The model under review builds one solid part; all positions refer to its coordinate system, in mm. A direction names the side the tool comes from. Coordinates: 2 decimals unless noted, no trailing zeros. Order: outer loops, then holes, each group sorted by start corner. A loop starts at its lowest first (then second) coordinate and runs counter-clockwise, first axis right, second up. Notation, with made-up numbers: (18, 26.25) -> (47, 26.25) arc R11 ccw to (47, 40.25) -> close; hole circle Ø11 at (69.5, 68). An arc over 180 degrees is marked (long way). Put each result on its own line as item: value.
from build123d import *

# Parameters (mm, degrees)
F0_R      = 22.5780805595
F5_DEPTH  = 25.4
F6_W      = 9.525
F6_H      = 38.1
F7_DEPTH  = 19.05
F8_R      = 5.08
F9_W      = 9.525
F9_H      = 38.1
F10_DEPTH = 19.05
F11_W     = 38.1
F11_H     = 9.525
F12_DEPTH = 19.05
F14_R     = 5.08
F13_W     = 8.255
F13_H     = 19.05
F15_DEPTH = 19.05
F16_R     = 8.25499
F17_SIZE  = 1.5875


# Not quite as in the source:
# - a fillet or chamfer is up to 0.001 mm smaller than in the source, because OpenCascade refuses the exact size


with BuildPart() as f2:
    # F2: sweep along a path in F1
    with BuildLine(Plane.XZ) as f2_path:
        Line((0, 0), (57.7025674284, 65.8432990313))
    # F0 (on Top) → F2 (sweep)
    with BuildSketch(Plane.XY):
        with Locations((-2.6368375402, 0)):
            Circle(F0_R)
    sweep(path=f2_path.line)


with BuildPart() as f5:
    # F4 (on Top) → F5 (new body)
    with BuildSketch(Plane.XY):
        with BuildLine():
            Line((-31.75, -19.05), (31.75, -19.05))
            Line((31.75, -19.05), (31.75, 19.05))
            Line((31.75, 19.05), (12.7, 19.05))
            ThreePointArc((12.7, 19.05), (0, 6.35), (-12.7, 19.05))
            Line((-12.7, 19.05), (-31.75, 19.05))
            Line((-31.75, 19.05), (-31.75, -19.05))
        make_face()
    extrude(amount=F5_DEPTH)

    # F6 (on face) → F7 (cut)
    with BuildSketch(Plane.XY.offset(25.4)):
        with Locations((26.9875, 0)):
            Rectangle(F6_W, F6_H)
    extrude(amount=-F7_DEPTH, mode=Mode.SUBTRACT)

    # F8
    f8_edges = [f5.edges().sort_by_distance(p)[0] for p in [
        (31.75, 19.05, 3.175),
    ]]
    fillet(f8_edges, radius=F8_R)

    # F9 (on face) → F10 (cut)
    with BuildSketch(Plane.XY.offset(25.4)):
        with Locations((-26.9875, 0)):
            Rectangle(F9_W, F9_H)
    extrude(amount=-F10_DEPTH, mode=Mode.SUBTRACT)

    # F11 (on face) → F12 (cut)
    with BuildSketch(Plane.XY.offset(25.4)):
        with Locations((0, -14.2875)):
            Rectangle(F11_W, F11_H)
    extrude(amount=-F12_DEPTH, mode=Mode.SUBTRACT)

    # F14
    f14_edges = [f5.edges().sort_by_distance(p)[0] for p in [
        (-31.75, 19.05, 3.175),
    ]]
    fillet(f14_edges, radius=F14_R)

    # F13 (on face) → F15 (cut)
    with BuildSketch(Plane.XY.offset(25.4)):
        with Locations((-18.0975, 9.525)):
            Rectangle(F13_W, F13_H)
        with Locations((18.0975, 9.525)):
            Rectangle(F13_W, F13_H)
    extrude(amount=-F15_DEPTH, mode=Mode.SUBTRACT)

    # F16 (radius 8.255 in the source; OpenCascade refuses exactly that, so slightly less here)
    f16_edges = [f5.edges().sort_by_distance(p)[0] for p in [
        (-13.97, 0, 15.875),
        (13.97, 0, 15.875),
    ]]
    fillet(f16_edges, radius=F16_R)

    # F17
    f17_edges = [f5.edges().sort_by_distance(p)[0] for p in [
        (0, 6.35, 25.4),
        (0, -9.525, 25.4),
        (-19.05, -14.2875, 25.4),
        (19.05, -14.2875, 25.4),
    ]]
    chamfer(f17_edges, length=F17_SIZE)


solid = f5.part
Item 1: For pin 1 Ø8.5 at (x, z) = (-4.5, 15) entering from -Y (3 decimals); pin 2 Ø7.5 at (y, z) = (-13, 13) entering from +X (3 decimals); pin 3 Ø2 at (x, z) = (-3, 19) entering from +Y, all flat-tipped, find the tip position at first contact; note any pin that passes through.
Answers below:
pin 1: y = -9.525
pin 2: x = 22.225
pin 3: y = 7
Item 2: For line 1 (X direction, y = -16.5, z = 10.25) (3 decimals); line 2 (Z direction, x = -8, y = -16); line 3 (X direction, y = -2, z = 7.75) (3 decimals), list the stretches that pass through material, from the lowest coordinate up. Write a range as from..to.
Answers below:
line 1: -22.225..-19.05, 19.05..22.225
line 2: 0..6.35
line 3: -22.225..22.225
Item 3: For faces 1 (the flat face through (25, 5, 6.35)), 2 (the flat face through (-25, 5, 6.35)), 3 (the flat face through (-22.225, -10, 16)), 4 (the flat face through (-19.05, -14, 15)), list the 3-axis set-ups (+Z, -Z, +X, -X, +Y, -Y) from which the entire face can be reached by the end or side of a thin tool; tool diameter is ignored.
Answers below:
face 1: +Z, +X, +Y
face 2: +Z, -X, +Y
face 3: +Z, -X, +Y, -Y
face 4: +Z, -Y
Item 4: Mouldability with a two-part tool opening along X and no side actions: class faces 5 (the flat face through (0, -9.525, 15)), 6 (the flat face through (0, -1, 25.4)), 7 (the cylindrical face through (30.301, 17.522, 3.219)) as +X half, -X half, draft (parallel to the pull), parting line (faces both ways), or undercut.
Answers below:
face 5: undercut
face 6: draft
face 7: +X half
Item 5: Consider section D-D on z = 4.5. Write out the cut boundary in (x, y), and give its area (3 significant figures).
Answers below:
outline: (-31.75, -19.05) -> (31.75, -19.05) -> (31.75, 13.97) arc R5.08 ccw to (26.67, 19.05) -> (12.7, 19.05) arc R12.7 cw to (-12.7, 19.05) -> (-26.67, 19.05) arc R5.08 ccw to (-31.75, 13.97) -> close
area: 2,150 mm^2
